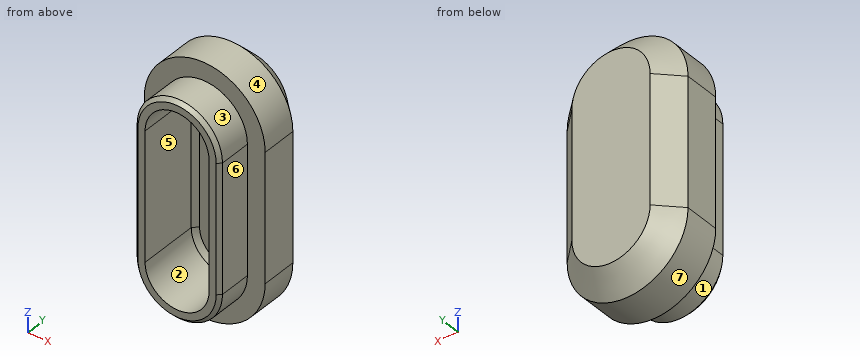
from build123d import *

# Parameters (mm, degrees)
EXTRUSION1_DEPTH = 8
CHANFREIN1_SIZE  = 3
COQUE1_T         = -4
EXTRUSION2_DEPTH = 5
CHANFREIN2_SIZE  = 0.5


with BuildPart() as part:
    # Esquisse1 → Extrusion1 (new body)
    with BuildSketch(Plane(origin=(0, 0, 0), x_dir=(1, 0, 0), z_dir=(0, 1, 0))):
        with BuildLine():
            Line((-8.5, 9), (-8.5, -9))
            ThreePointArc((-8.5, -9), (0, -17.5), (8.5, -9))
            Line((8.5, -9), (8.5, 9))
            ThreePointArc((8.5, 9), (0, 17.5), (-8.5, 9))
        make_face()
    extrude(amount=EXTRUSION1_DEPTH)

    # Chanfrein1
    chanfrein1_edges = [part.edges().sort_by_distance(p)[0] for p in [
        (0, 8, 17.5),
        (8.5, 8, 0),
        (0, 8, -17.5),
        (-8.5, 8, 0),
    ]]
    chamfer(chanfrein1_edges, length=CHANFREIN1_SIZE)

    # Coque1
    coque1_openings = [part.faces().sort_by_distance(p)[0] for p in [
        (0, 0, 0),
    ]]
    offset(amount=COQUE1_T, openings=coque1_openings, kind=Kind.INTERSECTION)

    # Esquisse2 → Extrusion2 (add)
    with BuildSketch(Plane.XZ):
        with BuildLine():
            Line((-6, -9), (-6, 9))
            ThreePointArc((-6, 9), (0, 15), (6, 9))
            Line((6, 9), (6, -9))
            ThreePointArc((6, -9), (0, -15), (-6, -9))
        make_face()
        with BuildLine():
            Line((4.5, 9), (4.5, -9))
            ThreePointArc((4.5, -9), (0, -13.5), (-4.5, -9))
            Line((-4.5, -9), (-4.5, 9))
            ThreePointArc((-4.5, 9), (0, 13.5), (4.5, 9))
        make_face(mode=Mode.SUBTRACT)
    extrude(amount=EXTRUSION2_DEPTH)

    # Chanfrein2
    chanfrein2_edges = [part.edges().sort_by_distance(p)[0] for p in [
        (0, -5, -15),
        (6, -5, 0),
        (0, -5, 15),
        (-6, -5, 0),
    ]]
    chamfer(chanfrein2_edges, length=CHANFREIN2_SIZE)


solid = part.part
CAD build for the part. Positions are in the model's coordinates, mm. Face numbers are marked on the shaded views. A direction names the side the tool comes from. Give positions to 0.01 mm unless a question says otherwise; leave off trailing zeros. Write each loop counter-clockwise with the first axis right and the second up, starting at its lowest first coordinate (ties: lowest second). Pieces come first, ordered by that corner, then holes. Notation, with made-up numbers: (82, 57.25) - (134, 57.25) arc R20 cw to (134, 90.25) - close; hole circle Ø4 at (-23, 53). An arc over 180 degrees is marked (long way). Answer as CSV lines item,"result".
Q1. Band-saw the part on D-D (y = 5.5). Give the cut face in (x, z), and give its area (3 significant figures).
Result set:
outline,"(-8, -9) arc R8 ccw to (8, -9) - (8, 9) arc R8 ccw to (-8, 9) - close"
area,"489 mm²"
Q2. 3-axis set-ups, long thin cutter, end or side, ignore diameter. For the marked faces 1, 2, 3 and 4: which of +Z, -Z, +X, -X, +Y, -Y reach the whole face in a straight line?
Result set:
face 1,"-Z, -Y"
face 2,"-Y"
face 3,"+Z, -Y"
face 4,"+Z, +Y, -Y"
Q3. Pull direction X, two halves, no side cores. Call the marked faces 5, 6 and 7: released by +X, released by -X, zero draft, split by the parting line, or undercut.
Result set:
face 5,"undercut"
face 6,"released by +X"
face 7,"split by the parting line"
Q4. Drill centre lines: line 1 (X direction, y = -1.5, z = 4.5); line 2 (X direction, y = 1.25, z = -0.5); line 3 (Y direction, x = 0.75, z = 2.5). Where is each one in solid material? Low to high. Write a range as from..to.
Result set:
line 1,"-6..-4.5, 4.5..6"
line 2,"-8.5..-4.5, 4.5..8.5"
line 3,"4..8"
Q5. Band-saw the part on C-C (x = 0). Give the cut face in (y, z).
Result set:
outline,"(-5, -14.5) - (-4.5, -15) - (0, -15) - (0, -17.5) - (5, -17.5) - (8, -14.5) - (8, 14.5) - (5, 17.5) - (0, 17.5) - (0, 15) - (-4.5, 15) - (-5, 14.5) - (-5, 13.5) - (3.34, 13.5) - (4, 12.84) - (4, -12.84) - (3.34, -13.5) - (-5, -13.5) - close"
Q6. Band-saw the part on A-A (y = 2). Give the cut face in (x, z).
Result set:
outline,"(-8.5, -9) arc R8.5 ccw to (8.5, -9) - (8.5, 9) arc R8.5 ccw to (-8.5, 9) - close; hole (-4.5, -9) arc R4.5 ccw to (4.5, -9) - (4.5, 9) arc R4.5 ccw to (-4.5, 9) - close"
Q7. Band-saw the part on B-B (z = 8). Give the cut face in (x, y).
Result set:
outline,"(-8.5, 0) - (-6, 0) - (-6, -4.5) - (-5.5, -5) - (-4.5, -5) - (-4.5, 3.34) - (-3.84, 4) - (3.84, 4) - (4.5, 3.34) - (4.5, -5) - (5.5, -5) - (6, -4.5) - (6, 0) - (8.5, 0) - (8.5, 5) - (5.5, 8) - (-5.5, 8) - (-8.5, 5) - close"
Q8. Flat gauge pins, fed straight in: pin 1 Ø1.3 at (y, z) = (-3, -3) entering from -X; pin 2 Ø6 at (x, z) = (6, -3) entering from -Y; pin 3 Ø2 at (x, z) = (1, 2) entering from -Y; pin 4 Ø4 at (x, y) = (6.5, 5) entering from -Z. Where does each tip first touch, or does it go through?
Result set:
pin 1,"x = -6"
pin 2,"y = -5"
pin 3,"y = 4"
pin 4,"z = -16.21"
